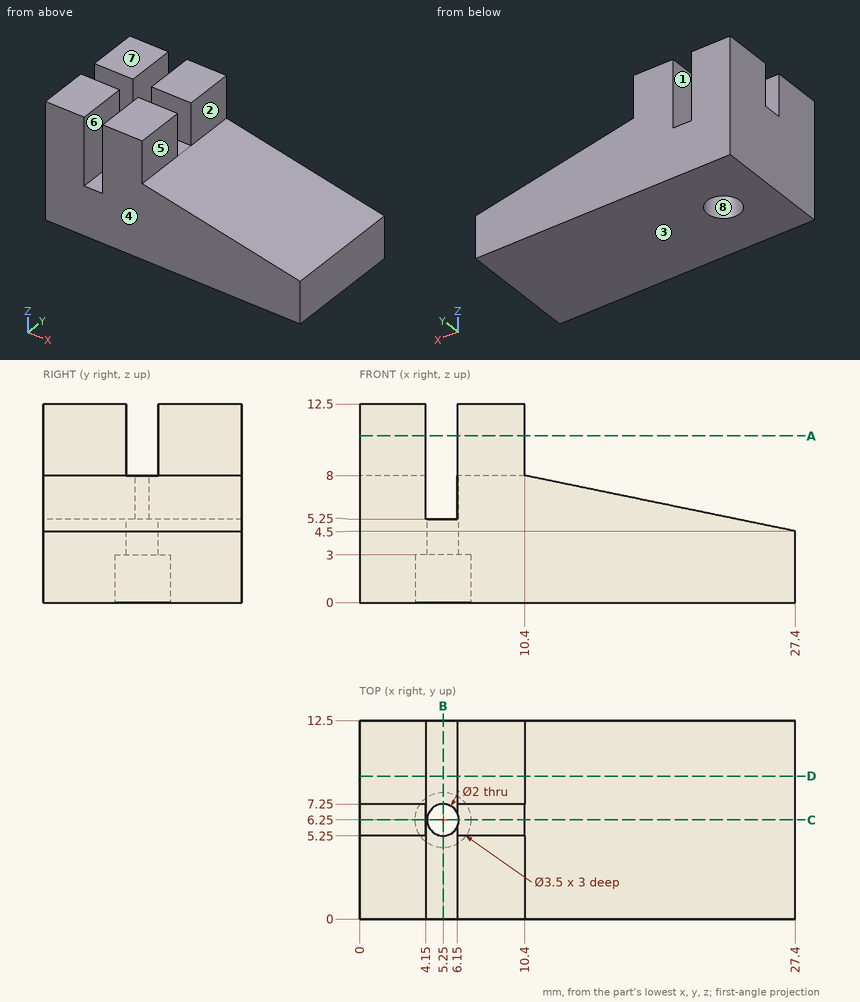
Job drawing, mm, ordinate dimensions from the low corner. One solid piece. A direction names the side the tool comes from. Give positions to 0.01 mm unless a question says otherwise; leave off trailing zeros. Write each loop counter-clockwise with the first axis right and the second up, starting at its lowest first coordinate (ties: lowest second). Pieces come first, ordered by that corner, then holes. Notation, with made-up numbers: M 73,52 L 132,52 A5 ccw 132,58 Z; hole C 59.25,15 d1. An arc over 180 degrees is marked long. One line per item, written item: value. Start each with the question number.
Q1. Two-plate mould, pull along X, no slides. Class the marked faces 1, 2 and 3: +X half, -X half, draft (parallel to the pull), parting line (faces both ways), or undercut.
Q2. Saw through at A-A, the plane z = 10.5. Write the cut outline in (x, y).
Q3. Drop flat-ended pins along their axis: pin 1 Ø1.3 at (y, z) = (2.5, 9) entering from +X; pin 2 Ø2.5 at (x, y) = (5.25, 6.25) entering from +Z; pin 3 Ø1 at (x, y) = (14, 11) entering from +Z. Give the stop position or say it passes through.
Q4. Saw through at B-B, the plane x = 5.25. Write the cut outline in (y, z), plus the area to 3 significant figures.
Q5. Probe probe 1 along X at (y, z) = (9.25, 8.75); probe 2 along Y at (x, z) = (5.25, 2.3); probe 3 along X at (y, z) = (6.25, 2.25). List the from-to ranges inside material, lowest first. Write a range as [from, to].
Q6. Saw through at D-D, the plane y = 9. Write the cut outline in (x, z), plus the area to 3 significant figures.
Q7. Saw through at C-C, the plane y = 6.25. Write the cut outline in (x, z), plus the area to 3 significant figures.
Q8. 3-axis set-ups, long thin cutter, end or side, ignore diameter. For the marked faces 4, 5, 6, 7 and 8: which of +Z, -Z, +X, -X, +Y, -Y reach the whole face in a straight line?
Output values:
1. face 1: undercut
1. face 2: +X half
1. face 3: draft
2. outline: M 0,0 L 4.15,0 L 4.15,5.25 L 0,5.25 Z; M 0,7.25 L 4.15,7.25 L 4.15,12.5 L 0,12.5 Z; M 6.15,0 L 10.4,0 L 10.4,5.25 L 6.15,5.25 Z; M 6.15,7.25 L 10.4,7.25 L 10.4,12.5 L 6.15,12.5 Z
3. pin 1: stops at x = 10.4
3. pin 2: stops at z = 8
3. pin 3: stops at z = 7.36
4. outline: M 0,0 L 4.5,0 L 4.5,3 L 5.25,3 L 5.25,5.25 L 0,5.25 Z; M 7.25,3 L 8,3 L 8,0 L 12.5,0 L 12.5,5.25 L 7.25,5.25 Z
4. area: 50.6 mm²
5. probe 1: x = [0, 4.15], [6.15, 10.4]
5. probe 2: y = [0, 4.5], [8, 12.5]
5. probe 3: x = [0, 3.5], [7, 27.4]
6. outline: M 0,0 L 27.4,0 L 27.4,4.5 L 10.4,8 L 10.4,12.5 L 6.15,12.5 L 6.15,5.25 L 4.15,5.25 L 4.15,12.5 L 0,12.5 Z
6. area: 222 mm²
7. outline: M 0,0 L 3.5,0 L 3.5,3 L 4.25,3 L 4.25,5.25 L 4.15,5.25 L 4.15,8 L 0,8 Z; M 6.25,3 L 7,3 L 7,0 L 27.4,0 L 27.4,4.5 L 10.4,8 L 6.25,8 Z
7. area: 169 mm²
8. face 4: +Z, -Z, +X, -X, -Y
8. face 5: +Z, +X, +Y, -Y
8. face 6: +Z, +Y, -Y
8. face 7: +Z, +X, -X, +Y, -Y
8. face 8: -Z
